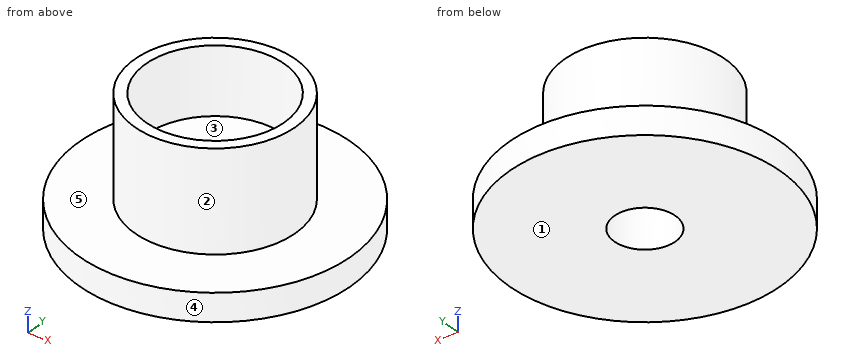
```python
from build123d import *

# Parameters (mm, degrees)
F0_R     = 24.5
F0_R_2   = 5.5
F1_DEPTH = 5
F2_R     = 14.5
F2_R_2   = 5.5
F3_DEPTH = 6
F4_R     = 12.5
F4_R_2   = 10
F4_R_3   = 14.5
F5_DEPTH = 12


with BuildPart() as f1:
    # F0 (on Top) → F1 (new body)
    with BuildSketch(Plane.XY):
        Circle(F0_R)
        Circle(F0_R_2, mode=Mode.SUBTRACT)
    extrude(amount=F1_DEPTH)

    # F2 (on face) → F3 (join)
    with BuildSketch(Plane.XY.offset(5)):
        Circle(F2_R)
        Circle(F2_R_2, mode=Mode.SUBTRACT)
    extrude(amount=F3_DEPTH)

    # F4 (on face) → F5 (join)
    with BuildSketch(Plane.XY.offset(11)):
        Circle(F4_R)
        Circle(F4_R_2, mode=Mode.SUBTRACT)
        Circle(F4_R_3)
        Circle(F4_R, mode=Mode.SUBTRACT)
    extrude(amount=F5_DEPTH)


solid = f1.part
```
CAD build for the part. Positions are in the model's coordinates, mm. Face numbers are marked on the shaded views. A direction names the side the tool comes from. Round coordinates to 2 decimals unless told otherwise and drop trailing zeros. Order: outer loops, then holes, each group sorted by start corner. A loop starts at its lowest first (then second) coordinate and runs counter-clockwise, first axis right, second up. Notation, with made-up numbers: (56, 48.5) - (93, 48.5) arc R15 cw to (93, 66.5) - close; hole circle Ø2 at (38.25, -13.75). An arc over 180 degrees is marked (long way). Use CSV: the item, a comma, the result in double quotes. Start each with the question number.
1) Tool access for the marked faces 4 and 5: list every direction of +Z, -Z, +X, -X, +Y, -Y with a clear straight run to the whole face (end or side of a thin tool).
2) Two-plate mould, pull along X, no slides. Class the marked faces 1, 2 and 3: pulls with the +X half, pulls with the -X half, needs draft (parallel to the pull), parting line crosses it, or undercut.
3) Wall check: L1, parallel to Y at x = 0, z = 6.5; L2, parallel to Z at x = 21, y = 5; L3, parallel to Y at x = -0.5, z = 16. Give the ranges that are in metal, low to high. Write a range as [from, to].
4) Saw through at C-C (z = 9.75). List the corners of the cut face in (x, y).
5) Saw through at D-D (x = 7.5). List the corners of the cut face in (y, z), and give its area (3 significant figures).
6) Pin check, flat tips, straight feed: pin 1 Ø10 at (y, z) = (-5.5, 7.5) entering from +X; pin 2 Ø3 at (x, z) = (-10.5, 14) entering from -Y; pin 3 Ø20 at (x, y) = (0, 0) entering from +Z. Stop position of each tip, or through.
7) Saw through at A-A (y = 0). List the corners of the cut face in (x, z).
Values follow:
1,face 4,"+Z, -Z"
1,face 5,"+Z"
2,face 1,"needs draft"
2,face 2,"parting line crosses it"
2,face 3,"undercut"
3,L1,"y = [-14.5, -5.5], [5.5, 14.5]"
3,L2,"z = [0, 5]"
3,L3,"y = [-14.49, -12.49], [12.49, 14.49]"
4,outline,"circle Ø29 at (0, 0); hole circle Ø11 at (0, 0)"
5,outline,"(-23.32, 0) - (23.32, 0) - (23.32, 5) - (12.41, 5) - (12.41, 23) - (10, 23) - (10, 11) - (-10, 11) - (-10, 23) - (-12.41, 23) - (-12.41, 5) - (-23.32, 5) - close"
5,area,"440 mm2"
6,pin 1,"stops at x = 24.47"
6,pin 2,"stops at y = -11.37"
6,pin 3,"stops at z = 11"
7,outline,"(-24.5, 0) - (-5.5, 0) - (-5.5, 11) - (-12.5, 11) - (-12.5, 23) - (-14.5, 23) - (-14.5, 5) - (-24.5, 5) - close; (5.5, 0) - (24.5, 0) - (24.5, 5) - (14.5, 5) - (14.5, 23) - (12.5, 23) - (12.5, 11) - (5.5, 11) - close"
